Design review of the part built by this model. Coordinates are the model's own, in mm. A direction names the side the tool comes from. Round coordinates to 2 decimals unless told otherwise and drop trailing zeros. Order: outer loops, then holes, each group sorted by start corner. A loop starts at its lowest first (then second) coordinate and runs counter-clockwise, first axis right, second up.
from build123d import *

# Parameters (mm, degrees)
SKETCH1_R           = 18
BOSS_EXTRUDE1_DEPTH = 110
SKETCH2_R           = 0.5
SKETCH3_R           = 11
BOSS_EXTRUDE2_DEPTH = 2
SKETCH4_R           = 4
BOSS_EXTRUDE3_DEPTH = 22
CUT_EXTRUDE1_START  = -15
CUT_EXTRUDE1_DEPTH  = 15
SKETCH6_R           = 5
BOSS_EXTRUDE4_DEPTH = 1
SKETCH7_R           = 2
CUT_EXTRUDE2_DEPTH  = 10


with BuildPart() as part:
    # Sketch1 → Boss-Extrude1 (new body)
    with BuildSketch(Plane.XY):
        Circle(SKETCH1_R)
    extrude(amount=BOSS_EXTRUDE1_DEPTH)

    # Sketch2 → Cut-Revolve1 (revolve, cut)
    with BuildSketch(Plane(origin=(0, 0, 0), x_dir=(1, 0, 0), z_dir=(0, 1, 0)), mode=Mode.PRIVATE) as cut_revolve1_sk:
        with Locations((18, -57)):
            Circle(SKETCH2_R)
    revolve(cut_revolve1_sk.sketch.rotate(Axis((0, 0, 0), (0, 0, 1)), 180), axis=Axis((0, 0, 0), (0, 0, 1)), mode=Mode.SUBTRACT)

    # Sketch3 → Boss-Extrude2 (add)
    with BuildSketch(Plane.XY.offset(110)):
        Circle(SKETCH3_R)
    extrude(amount=BOSS_EXTRUDE2_DEPTH)

    # Sketch4 → Boss-Extrude3 (add)
    with BuildSketch(Plane.XY.offset(112)):
        Circle(SKETCH4_R)
    extrude(amount=BOSS_EXTRUDE3_DEPTH)

    # Sketch5 → Cut-Extrude1 (cut)
    with BuildSketch(Plane.XY.offset(134).offset(CUT_EXTRUDE1_START)):
        with BuildLine():
            Line((-1.936491673, -3.5), (1.936491673, -3.5))
            ThreePointArc((1.936491673, -3.5), (0, -4), (-1.936491673, -3.5))
        make_face()
    extrude(amount=CUT_EXTRUDE1_DEPTH, mode=Mode.SUBTRACT)

    # Sketch6 → Boss-Extrude4 (add)
    with BuildSketch(Plane(origin=(0, 0, 0), x_dir=(-1, 0, 0), z_dir=(0, 0, -1))):
        Circle(SKETCH6_R)
    extrude(amount=BOSS_EXTRUDE4_DEPTH)

    # Sketch7 → Cut-Extrude2 (cut)
    with BuildSketch(Plane.XY.offset(110)):
        with Locations((14, 0)):
            Circle(SKETCH7_R)
        with Locations((0, -14)):
            Circle(SKETCH7_R)
        with Locations((-14, 0)):
            Circle(SKETCH7_R)
        with Locations((0, 14)):
            Circle(SKETCH7_R)
    extrude(amount=-CUT_EXTRUDE2_DEPTH, mode=Mode.SUBTRACT)


solid = part.part
1) To check wall thickness, follow line 1 along Y through (x, z) = (0, 102); line 2 along Z through (x, y) = (10.5, 0.5); line 3 along Z through (x, y) = (-13.5, -1). State the ranges of each line that lie inside material, in increasing order.
Results:
line 1: y = -18 to -16, -12 to 12, 16 to 18
line 2: z = 0 to 112
line 3: z = 0 to 100
2) For faces 1 (the face through (-0.521, 3.966, 122.846)), 2 (the face through (4, -4, 0)), 3 (the face through (0, -3.5, 126)), list the 3-axis set-ups (+Z, -Z, +X, -X, +Y, -Y) from which the entire face can be reached by the end or side of a thin tool; tool diameter is ignored.
Results:
face 1: +Z
face 2: -Z
face 3: +Z, +X, -X, -Y
3) Take a section at C-C on z = 31. Give the boundary of the cut face in (x, y), plus the area to 3 significant figures.
Results:
outline: circle Ø36 at (0, 0)
area: 1,020 mm2
4) The part is to be moulded in two halves that separate along Y. For faces 4 (the face through (-2.343, 17.847, 27.854)), 5 (the face through (12.4, -1.2, 105.1)), 6 (the face through (-8, -8, 110)), say which applies: released by +Y, released by -Y, zero draft, split by the parting line, or undercut.
Results:
face 4: split by the parting line
face 5: undercut
face 6: zero draft
5) Take a section at A-A on y = 0. Give the boundary of the cut face in (x, z), plus the area to 3 significant figures.
Results:
outline: (-18, 0) - (-5, 0) - (-5, -1) - (5, -1) - (5, 0) - (18, 0) - (18, 56.5) arc R0.5 cw to (18, 57.5) - (18, 110) - (16, 110) - (16, 100) - (12, 100) - (12, 110) - (11, 110) - (11, 112) - (4, 112) - (4, 134) - (-4, 134) - (-4, 112) - (-11, 112) - (-11, 110) - (-12, 110) - (-12, 100) - (-16, 100) - (-16, 110) - (-18, 110) - (-18, 57.5) arc R0.5 cw to (-18, 56.5) - close
area: 4,110 mm2
6) Clearance check with flat-ended pins moving along their axes: P1, Ø1, axis at y = 1, z = 36, coming from the +X side; P2, Ø4, axis at y = -12.5, z = 72, coming from the +X side; P3, Ø1.2, axis at x = 0, y = 13, coming from the +Z side. State where each tip first meets the part, or that it passes through.
Results:
P1: stops at x = 17.99
P2: stops at x = 14.62
P3: stops at z = 100
